The listing builds one solid part. Answer for the finished solid, in the listing's coordinates (mm). A direction names the side the tool comes from. Round coordinates to 2 decimals unless told otherwise and drop trailing zeros. Write each loop counter-clockwise with the first axis right and the second up, starting at its lowest first coordinate (ties: lowest second). Pieces come first, ordered by that corner, then holes. Notation, with made-up numbers: (-21.75, 13.5) - (-8.75, 13.5) arc R15 cw to (-8.75, 42.5) - close; hole circle Ø1 at (55, 59.25). An arc over 180 degrees is marked (long way). Return JSON: item names as keys, results as strings. Group by question number.
from build123d import *

# Parameters (mm, degrees)
SKETCH_1_W          = 100
SKETCH_1_H          = 7
EXTRUDE_1_DEPTH     = 5
SKETCH_2_R          = 1.1
CUT_EXTRUDE_1_DEPTH = 101.369318021
SKETCH_3_W          = 30
SKETCH_3_H          = 20
EXTRUDE_2_DEPTH     = 5
SKETCH_4_W          = 5
SKETCH_4_H          = 7
EXTRUDE_3_DEPTH     = 15
SKETCH_5_R          = 1.65
CUT_EXTRUDE_2_DEPTH = 15
FILLET_1_R          = 5


with BuildPart() as part:
    # 草图1 → 凸台-拉伸1 (new body)
    with BuildSketch(Plane.XY):
        with Locations((50, 3.5)):
            Rectangle(SKETCH_1_W, SKETCH_1_H)
    extrude(amount=EXTRUDE_1_DEPTH)

    # 草图2 → 切除-拉伸1 (cut, through all)
    with BuildSketch(Plane(origin=(0, 0, 0), x_dir=(-1, 0, 0), z_dir=(0, 0, -1))):
        with Locations((-95, 3.5)):
            Circle(SKETCH_2_R)
        with Locations((-80, 3.5)):
            Circle(SKETCH_2_R)
        with Locations((-65, 3.5)):
            Circle(SKETCH_2_R)
        with Locations((-50, 3.5)):
            Circle(SKETCH_2_R)
        with Locations((-35, 3.5)):
            Circle(SKETCH_2_R)
        with Locations((-20, 3.5)):
            Circle(SKETCH_2_R)
        with Locations((-5, 3.5)):
            Circle(SKETCH_2_R)
    extrude(amount=-CUT_EXTRUDE_1_DEPTH, mode=Mode.SUBTRACT)

    # 草图3 → 凸台-拉伸2 (add)
    with BuildSketch(Plane(origin=(0, 0, 0), x_dir=(-1, 0, 0), z_dir=(0, 0, -1))):
        with Locations((-85, -10)):
            Rectangle(SKETCH_3_W, SKETCH_3_H)
    extrude(amount=-EXTRUDE_2_DEPTH)

    # 草图4 → 凸台-拉伸3 (add)
    with BuildSketch(Plane.XY.offset(5)):
        with Locations((-2.5, 3.5)):
            Rectangle(SKETCH_4_W, SKETCH_4_H)
    extrude(amount=-EXTRUDE_3_DEPTH)

    # 草图5 → 切除-拉伸2 (cut)
    with BuildSketch(Plane(origin=(0, 0, 0), x_dir=(-1, 0, 0), z_dir=(0, 0, -1))):
        with Locations((-95, -14.9)):
            Circle(SKETCH_5_R)
        with Locations((-75, -14.9)):
            Circle(SKETCH_5_R)
    extrude(amount=-CUT_EXTRUDE_2_DEPTH, mode=Mode.SUBTRACT)

    # 圆角1
    fillet_1_edges = [part.edges().sort_by_distance(p)[0] for p in [
        (70, 0, 2.5),
        (100, 7, 2.5),
    ]]
    fillet(fillet_1_edges, radius=FILLET_1_R)


solid = part.part
(1) Find section A-A (x = 80). Write down the section's boundary in (y, z), plus the area to 3 significant figures.
(2) Find section C-C (z = -8.75). Write down the section's boundary in (x, y).
(3) For faces 1 (the cylindrical face through (76.31, -15.9, 2.46)), 2 (the flat face through (70, -13, 2)), 3 (the flat face through (73, -3, 0)), determine the directions among +Z, -Z, +X, -X, +Y, -Y from which every point of the face is accessible in a straight line to the end or side of a thin tool.
(4) Flat-ended cylindrical pins translate along their axes: pin 1 (4 mm diameter, centred on x = 75, y = -14.9, fed in from -Z); pin 2 (4 mm diameter, centred on y = -9, z = 2, fed in from -X); pin 3 (5.5 mm diameter, centred on y = 2.5, z = -6, fed in from +X). Find the tip coordinate at first contact, or state that the pin passes through.
(5) Find section D-D (x = 35). Write down the section's boundary in (y, z).
(6) Find section B-B (y = -14.9). Write down the section's boundary in (x, z), plus the area to 3 significant figures.
(7) Consider line 1 (Y direction, x = 5, z = 1.75); line 2 (Y direction, x = 95, z = 3.8); line 3 (X direction, y = -15.25, z = 0.5). Determine where each line is inside the solid, lowest interval first.
(8) Determine the mould class of faces 4 (the flat face through (22, 0, 1)), 5 (the flat face through (100, -9, 2)), 6 (the cylindrical face through (81.1, 3.5, 2.5)) for opening direction Y: +Y half, -Y half, draft (parallel to the pull), parting line (faces both ways), or undercut.
Check sheet entries:
{
 "1": {"outline": "(-20, 0) - (2.4, 0) - (2.4, 5) - (-20, 5) - close; (4.6, 0) - (7, 0) - (7, 5) - (4.6, 5) - close", "area": "124 mm^2"},
 "2": {"outline": "(-5, 0) - (0, 0) - (0, 7) - (-5, 7) - close"},
 "3": {"face 1": "+Z, -Z", "face 2": "+Z, -Z, -X, -Y", "face 3": "-Z, +X, +Y, -Y"},
 "4": {"pin 1": "stops at z = 0", "pin 2": "stops at x = 70", "pin 3": "stops at x = 0"},
 "5": {"outline": "(0, 0) - (2.4, 0) - (2.4, 5) - (0, 5) - close; (4.6, 0) - (7, 0) - (7, 5) - (4.6, 5) - close"},
 "6": {"outline": "(70, 0) - (73.35, 0) - (73.35, 5) - (70, 5) - close; (76.65, 0) - (93.35, 0) - (93.35, 5) - (76.65, 5) - close; (96.65, 0) - (100, 0) - (100, 5) - (96.65, 5) - close", "area": "117 mm^2"},
 "7": {"line 1": "y = 0 to 2.4, 4.6 to 7", "line 2": "y = -20 to -16.55, -13.25 to 2.4, 4.6 to 7", "line 3": "x = 70 to 73.39, 76.61 to 93.39, 96.61 to 100"},
 "8": {"face 4": "-Y half", "face 5": "draft", "face 6": "undercut"}
}
